Geometry check sheet. Reference: the model listing, model coordinates, mm. Round coordinates to 2 decimals unless told otherwise and drop trailing zeros. Write each loop counter-clockwise with the first axis right and the second up, starting at its lowest first coordinate (ties: lowest second). Pieces come first, ordered by that corner, then holes. Notation, with made-up numbers: (16.5, -23) -> (74.5, -23) arc R25 cw to (74.5, -10) -> close; hole circle Ø7 at (32, -29.75). An arc over 180 degrees is marked (long way). Use a Markdown table: item, result.
```python
from build123d import *

# Parameters (mm, degrees)
SKETCH1_R           = 2.38125
BOSS_EXTRUDE1_DEPTH = 1.5875


with BuildPart() as part:
    # Sketch1 → Boss-Extrude1 (new body)
    with BuildSketch(Plane(origin=(0, 0, 0), x_dir=(1, 0, 0), z_dir=(0, 1, 0))):
        with BuildLine():
            Line((-25.4, -6.35), (25.4, -6.35))
            ThreePointArc((25.4, -6.35), (31.75, 0), (25.4, 6.35))
            Line((25.4, 6.35), (-25.4, 6.35))
            ThreePointArc((-25.4, 6.35), (-31.75, 0), (-25.4, -6.35))
        make_face()
        with Locations((-25.4, 0)):
            Circle(SKETCH1_R, mode=Mode.SUBTRACT)
        with Locations((-12.7, 0)):
            Circle(SKETCH1_R, mode=Mode.SUBTRACT)
        Circle(SKETCH1_R, mode=Mode.SUBTRACT)
        with Locations((12.7, 0)):
            Circle(SKETCH1_R, mode=Mode.SUBTRACT)
        with Locations((25.4, 0)):
            Circle(SKETCH1_R, mode=Mode.SUBTRACT)
    extrude(amount=BOSS_EXTRUDE1_DEPTH)


solid = part.part
```
(1) Section check D-D on x = 14. Record the cut outline in (y, z), plus the area to 3 significant figures.
A:
| item | result |
|---|---|
| outline | (0, -6.35) -> (1.59, -6.35) -> (1.59, -2) -> (0, -2) -> close; (0, 2) -> (1.59, 2) -> (1.59, 6.35) -> (0, 6.35) -> close |
| area | 13.8 mm2 |
(2) Thickness scan on line 1 (X direction, y = 1, z = 0); line 2 (Z direction, x = -12.7, y = 0.45); line 3 (X direction, y = 0.45, z = 2). Record the ranges inside material, lowest first.
A:
| item | result |
|---|---|
| line 1 | x = -31.75 to -27.78, -23.02 to -15.08, -10.32 to -2.38, 2.38 to 10.32, 15.08 to 23.02, 27.78 to 31.75 |
| line 2 | z = -6.35 to -2.38, 2.38 to 6.35 |
| line 3 | x = -31.43 to -26.69, -24.11 to -13.99, -11.41 to -1.29, 1.29 to 11.41, 13.99 to 24.11, 26.69 to 31.43 |
(3) Release check for a two-part mould opening along X. For faces 1 (the face through (-27.78, 0.78, -0.1)), 2 (the face through (0, 1.588, -3)), 3 (the face through (-31.75, 0.78, -0.14)) record: +X half, -X half, draft (parallel to the pull), parting line (faces both ways), or undercut.
A:
| item | result |
|---|---|
| face 1 | undercut |
| face 2 | draft |
| face 3 | -X half |
(4) Section check B-B on x = 0. Record the cut outline in (y, z), plus the area to 3 significant figures.
A:
| item | result |
|---|---|
| outline | (0, -6.35) -> (1.59, -6.35) -> (1.59, -2.38) -> (0, -2.38) -> close; (0, 2.38) -> (1.59, 2.38) -> (1.59, 6.35) -> (0, 6.35) -> close |
| area | 12.6 mm2 |
(5) Section check A-A on z = 0. Record the cut outline in (x, y), plus the area to 3 significant figures.
A:
| item | result |
|---|---|
| outline | (-31.75, 0) -> (-27.78, 0) -> (-27.78, 1.59) -> (-31.75, 1.59) -> close; (-23.02, 0) -> (-15.08, 0) -> (-15.08, 1.59) -> (-23.02, 1.59) -> close; (-10.32, 0) -> (-2.38, 0) -> (-2.38, 1.59) -> (-10.32, 1.59) -> close; (2.38, 0) -> (10.32, 0) -> (10.32, 1.59) -> (2.38, 1.59) -> close; (15.08, 0) -> (23.02, 0) -> (23.02, 1.59) -> (15.08, 1.59) -> close; (27.78, 0) -> (31.75, 0) -> (31.75, 1.59) -> (27.78, 1.59) -> close |
| area | 63.0 mm2 |
(6) Section check C-C on y = 1.15. Record the cut outline in (x, z).
A:
| item | result |
|---|---|
| outline | (-25.4, -6.35) -> (25.4, -6.35) arc R6.35 ccw to (25.4, 6.35) -> (-25.4, 6.35) arc R6.35 ccw to start; hole circle Ø4.76 at (-25.4, 0); hole circle Ø4.76 at (-12.7, 0); hole circle Ø4.76 at (0, 0); hole circle Ø4.76 at (12.7, 0); hole circle Ø4.76 at (25.4, 0) |
